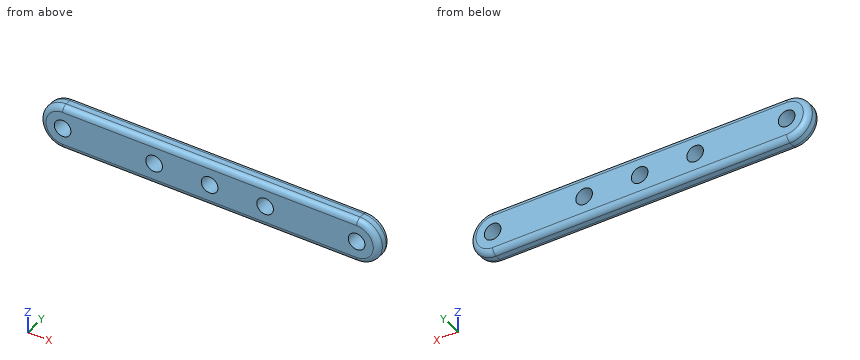
```python
from build123d import *

# Parameters (mm, degrees)
SKETCH1_R           = 1.5
BOSS_EXTRUDE1_DEPTH = 3
FILLET1_R           = 1


with BuildPart() as part:
    # Sketch1 → Boss-Extrude1 (new body)
    with BuildSketch(Plane(origin=(0, 0, 0), x_dir=(1, 0, 0), z_dir=(0, 1, 0))):
        with BuildLine():
            Line((-26.5, 4), (26.5, 4))
            ThreePointArc((26.5, 4), (30.5, 0), (26.5, -4))
            Line((26.5, -4), (-26.5, -4))
            ThreePointArc((-26.5, -4), (-30.5, 0), (-26.5, 4))
        make_face()
        with Locations((-26.5, 0)):
            Circle(SKETCH1_R, mode=Mode.SUBTRACT)
        with Locations((26.5, 0)):
            Circle(SKETCH1_R, mode=Mode.SUBTRACT)
        with Locations((-10, 0)):
            Circle(SKETCH1_R, mode=Mode.SUBTRACT)
        with Locations((10, 0)):
            Circle(SKETCH1_R, mode=Mode.SUBTRACT)
        Circle(SKETCH1_R, mode=Mode.SUBTRACT)
    extrude(amount=BOSS_EXTRUDE1_DEPTH)

    # Fillet1
    fillet1_edges = [part.edges().sort_by_distance(p)[0] for p in [
        (30.5, 0, 0),
        (0, 0, 4),
        (-30.5, 0, 0),
        (0, 0, -4),
        (0, 3, -4),
        (-30.5, 3, 0),
        (0, 3, 4),
        (30.5, 3, 0),
    ]]
    fillet(fillet1_edges, radius=FILLET1_R)


solid = part.part
```
The listing builds one solid part. Answer for the finished solid, in the listing's coordinates (mm). Coordinates: 2 decimals unless noted, no trailing zeros. Write each loop counter-clockwise with the first axis right and the second up, starting at its lowest first coordinate (ties: lowest second). Pieces come first, ordered by that corner, then holes. Notation, with made-up numbers: M 28.5,33 L 69.5,33 A12 ccw 69.5,48 Z; hole C 38,5.5 d6. An arc over 180 degrees is marked long. Use a Markdown table: item, result. Add a question column.
1. Straight lines are drawn through the part: line 1 along X through (y, z) = (1.5, 0); line 2 along Z through (x, y) = (10, 1); line 3 along X through (y, z) = (2.35, 0). For each, find the intervals that lie inside material, in ascending order. Write a range as [from, to].
2. Section A-A (y = 1.5) is taken. Give the vertices of the cut face in (x, z), plus the area to 3 significant figures.
3. Section D-D (z = 0.75) is taken. Count the separate pieces of the cut face and the enclosed holes in it, plus the area to 3 significant figures.
4. Section B-B (x = 0) is taken. Give the vertices of the cut face in (y, z), plus the area to 3 significant figures.
5. Section C-C (x = 7) is taken. Give the vertices of the cut face in (y, z).
Data:
| question | item | result |
|---|---|---|
| 1 | line 1 | x = [-30.5, -28], [-25, -11.5], [-8.5, -1.5], [1.5, 8.5], [11.5, 25], [28, 30.5] |
| 1 | line 2 | z = [-4, -1.5], [1.5, 4] |
| 1 | line 3 | x = [-30.44, -28], [-25, -11.5], [-8.5, -1.5], [1.5, 8.5], [11.5, 25], [28, 30.44] |
| 2 | outline | M -26.5,-4 L 26.5,-4 A4 ccw 26.5,4 L -26.5,4 A4 ccw Z; hole C -26.5,0 d3; hole C -10,0 d3; hole C 0,0 d3; hole C 10,0 d3; hole C 26.5,0 d3 |
| 2 | area | 439 mm2 |
| 3 | separate pieces | 6 |
| 3 | enclosed holes | 0 |
| 3 | area | 143 mm2 |
| 4 | outline | M 0,-3 A1 ccw 1,-4 L 2,-4 A1 ccw 3,-3 L 3,-1.5 L 0,-1.5 Z; M 0,1.5 L 3,1.5 L 3,3 A1 ccw 2,4 L 1,4 A1 ccw 0,3 Z |
| 4 | area | 14.1 mm2 |
| 5 | outline | M 0,-3 A1 ccw 1,-4 L 2,-4 A1 ccw 3,-3 L 3,3 A1 ccw 2,4 L 1,4 A1 ccw 0,3 Z |
